from build123d import *

# Parameters (mm, degrees)
F1_DEPTH = 5


with BuildPart() as f1:
    # F0 (on Top) → F1 (new body, symmetric)
    with BuildSketch(Plane.XY):
        with BuildLine():
            Line((7.5, 29.233247), (-7.5, 29.233247))
            Line((-7.5, 29.233247), (-7.5, 4.45))
            ThreePointArc((-7.5, 4.45), (-4.353375, 3.146625), (-3.05, 0))
            ThreePointArc((-3.05, 0), (-4.353375, -3.146625), (-7.5, -4.45))
            Line((-7.5, -4.45), (-7.5, -29.233247))
            Line((-7.5, -29.233247), (7.5, -29.233247))
            Line((7.5, -29.233247), (7.5, -4.45))
            ThreePointArc((7.5, -4.45), (3.05, 0), (7.5, 4.45))
            Line((7.5, 4.45), (7.5, 29.233247))
        make_face()
        with BuildLine():
            Line((-7.5, 4.45), (-7.5, 29.233247))
            Line((-7.5, 29.233247), (-22.5, 29.233247))
            Line((-22.5, 29.233247), (-22.5, -35.766753))
            Line((-22.5, -35.766753), (-7.5, -35.766753))
            Line((-7.5, -35.766753), (-7.5, -29.233247))
            Line((-7.5, -29.233247), (-7.5, -4.45))
            ThreePointArc((-7.5, -4.45), (-11.95, 0), (-7.5, 4.45))
        make_face()
        with BuildLine():
            Line((22.5, 29.233247), (7.5, 29.233247))
            Line((7.5, 29.233247), (7.5, 4.45))
            ThreePointArc((7.5, 4.45), (10.646625, 3.146625), (11.95, 0))
            ThreePointArc((11.95, 0), (10.646625, -3.146625), (7.5, -4.45))
            Line((7.5, -4.45), (7.5, -29.233247))
            Line((7.5, -29.233247), (7.5, -35.766753))
            Line((7.5, -35.766753), (22.5, -35.766753))
            Line((22.5, -35.766753), (22.5, 29.233247))
        make_face()
    extrude(amount=F1_DEPTH, both=True)


solid = f1.part
The model under review builds one solid part; all positions refer to its coordinate system, in mm. A direction names the side the tool comes from. Round coordinates to 2 decimals unless told otherwise and drop trailing zeros. Loops run counter-clockwise (first coordinate to the right, second up) from the corner with the lowest first, then second, coordinate; pieces in that order, holes last. Notation, with made-up numbers: M 67.25,31.25 L 100.25,31.25 A24 ccw 100.25,59.25 Z; hole C -22,68 d9. An arc over 180 degrees is marked long. Answer as a JSON object with one key per item and string values.
Item 1: The part is to be moulded in two halves that separate along X. For faces 3 (the face through (-7.5, -33, 0)), 4 (the face through (15, -35.767, 0)), 5 (the face through (0, -29.233, 0)), 6 (the face through (-22.5, -3, 0)), say which applies: +X half, -X half, draft (parallel to the pull), parting line (faces both ways), or undercut.
Check sheet entries:
{"face 3": "undercut", "face 4": "draft", "face 5": "undercut", "face 6": "-X half"}
Item 2: For line 1 along X through (y, z) = (3, -4); line 2 along Y through (x, z) = (1, 2); line 3 along Y through (x, z) = (6, 1.5), list the stretches that pass through material, from the lowest coordinate up.
Check sheet entries:
{"line 1": "-22.5 to -10.79, -4.21 to 4.21, 10.79 to 22.5", "line 2": "-29.23 to 29.23", "line 3": "-29.23 to -4.19, 4.19 to 29.23"}
Item 3: We need section C-C, the plane x = 4. State the section outline as (y, z) points, and give its area (3 significant figures).
Check sheet entries:
{"outline": "M -29.23,-5 L -2.75,-5 L -2.75,5 L -29.23,5 Z; M 2.75,-5 L 29.23,-5 L 29.23,5 L 2.75,5 Z", "area": "530 mm2"}
Item 4: Tool access review of faces 1 (the face through (-15, -35.767, 0)), 2 (the face through (7.5, -32, 0)): name each direction out of +Z, -Z, +X, -X, +Y, -Y from which nothing blocks a thin tool from reaching the whole face with its end or side.
Check sheet entries:
{"face 1": "+Z, -Z, +X, -X, -Y", "face 2": "+Z, -Z, -Y"}
Item 5: We need section A-A, the plane z = -0.5. State the section outline as (x, y) points.
Check sheet entries:
{"outline": "M -22.5,-35.77 L -7.5,-35.77 L -7.5,-29.23 L 7.5,-29.23 L 7.5,-35.77 L 22.5,-35.77 L 22.5,29.23 L -22.5,29.23 Z; hole M -7.5,4.45 A4.45 ccw long -3.05,0 A4.45 ccw Z; hole M 7.5,4.45 A4.45 ccw long 11.95,0 A4.45 ccw Z"}
Item 6: We need section B-B, the plane x = -4.5. State the section outline as (y, z) points.
Check sheet entries:
{"outline": "M -29.23,-5 L -3.29,-5 L -3.29,5 L -29.23,5 Z; M 3.29,-5 L 29.23,-5 L 29.23,5 L 3.29,5 Z"}
Item 7: Clearance check with a flat-ended pin moving along its axis: P1, Ø5, axis at x = 0.5, z = 0, coming from the -Y side. State where the tip first meets the part, or that it passes through.
Check sheet entries:
{"P1": "y = -29.23"}
